Verification items for the finished model (mm, model axes). A direction names the side the tool comes from. Give positions to 0.01 mm unless a question says otherwise; leave off trailing zeros. Order: outer loops, then holes, each group sorted by start corner. A loop starts at its lowest first (then second) coordinate and runs counter-clockwise, first axis right, second up. Notation, with made-up numbers: (-24.5, 77) -> (15.5, 77) arc R10 cw to (15.5, 91) -> close; hole circle Ø11 at (-21.75, 83.25). An arc over 180 degrees is marked (long way). Return JSON: item names as keys, results as strings. Group by question number.
(1) Tool access check on faces 4 (the face through (-18, 0, 12.3)), 5 (the face through (-0.3, -18, 9.8)), 6 (the face through (0.3, 18, 9.8)). Record the directions out of +Z, -Z, +X, -X, +Y, -Y that give a thin tool (end or side, any length) a straight path to the whole face; none if there is none.
(2) Cross-section at C-C on x = 8. Enter the section's corners in (y, z).
(3) Depth check by flat-ended pin: pin 1 Ø5.5 at (x, y) = (6, 27) entering from -Z; pin 2 Ø3.5 at (x, y) = (-18, 7) entering from +Z; pin 3 Ø8.5 at (x, y) = (0, 0) entering from +Z; pin 4 Ø3 at (x, z) = (-10.5, 10) entering from -Y. Enter the tip coordinate at first touch or a pass-through.
(4) Thickness scan on line 1 along X through (y, z) = (0, 14.2); line 2 along X through (y, z) = (0, 9.55); line 3 along Y through (x, z) = (0, 13.1). Record the ranges inside material, lowest first.
(5) Cross-section at B-B on z = 15.5. Enter the section's corners in (x, y), then the cut area to 3 significant figures.
(6) Cross-section at A-A on x = 0. Enter the section's corners in (y, z).
(7) Release check for a two-part mould opening along Y. For faces 1 (the face through (0, -35, 14)), 2 (the face through (3, -2, 10.8)), 3 (the face through (15, 34, 14)) record: pulls with the +Y half, pulls with the -Y half, needs draft (parallel to the pull), parting line crosses it, or undercut.
Autodesk Fusion 360 part; units mm, degrees
ref_plane "工作平面1" through (0, 0, 12.3) normal (0, 0, 1) x (1, 0, 0)
sketch "草图1" plane through (0, 0, 12.3) normal (0, 0, 1) x (1, 0, 0)
  line L0 (-33, -16) -> (33, -16)
  line L1 (33, -16) -> (35, -14)
  line L2 (35, -14) -> (35, 14)
  line L3 (35, 14) -> (33, 16)
  line L4 (33, 16) -> (-33, 16)
  line L5 (-33, 16) -> (-35, 14)
  line L6 (-35, 14) -> (-35, -14)
  line L7 (-35, -14) -> (-33, -16)
extrude "70 x 32 camera support plate" add sketch "草图1" along normal blind 4
ref_plane "工作平面2" through (0, 0, 7.3) normal (0, 0, 1) x (1, 0, 0)
sketch "草图2" plane through (0, 0, 7.3) normal (0, 0, 1) x (1, 0, 0)
  line L0 (-20, -19) -> (20, -19)
  line L1 (20, -19) -> (20, 19)
  line L2 (20, 19) -> (-20, 19)
  line L3 (-20, 19) -> (-20, -19)
ref_plane "工作平面3" through (0, 0, 12.3) normal (0, 0, 1) x (1, 0, 0)
sketch "草图3" plane through (0, 0, 12.3) normal (0, 0, 1) x (1, 0, 0)
  line L0 (-16, -19) -> (16, -19)
  line L1 (16, -19) -> (16, 19)
  line L2 (16, 19) -> (-16, 19)
  line L3 (-16, 19) -> (-16, -19)
loft "40 to 32 mm male dovetail" add profiles "草图2", "草图3" section 1 section 2
ref_plane "工作平面4" through (0, 0, 7.3) normal (0, 0, 1) x (1, 0, 0)
sketch "草图4" plane through (0, 0, 7.3) normal (0, 0, 1) x (1, 0, 0)
  circle A0 centre (0, 0) radius 3.4
extrude "1/4 inch metal screw clearance 6.8 mm" cut sketch "草图4" along normal blind 9
ref_plane "工作平面5" through (0, 0, 7.3) normal (0, 0, 1) x (1, 0, 0)
sketch "草图5" plane through (0, 0, 7.3) normal (0, 0, 1) x (1, 0, 0)
  circle A0 centre (0, 0) radius 7
extrude "14 x 3.5 mm screw head recess" cut sketch "草图5" along normal blind 3.5
move_body "Align camera long edge with gimbal arm - 90 degrees" bodies 1 to x (0, 1, 0) y (-1, 0, 0) z (0, 0, 1) at (0, 0, 0)
Verdict:
{
 "1": {"face 4": "+Z, -X, +Y, -Y", "face 5": "+X, -X, -Y", "face 6": "+X, -X, +Y"},
 "2": {"outline": "(-35, 12.3) -> (-16, 12.3) -> (-20, 7.3) -> (20, 7.3) -> (16, 12.3) -> (35, 12.3) -> (35, 16.3) -> (-35, 16.3) -> close"},
 "3": {"pin 1": "z = 12.3", "pin 2": "z = 12.3", "pin 3": "z = 16.3", "pin 4": "y = -19.04"},
 "4": {"line 1": "-16 to -3.4, 3.4 to 16", "line 2": "-19 to -7, 7 to 19", "line 3": "-35 to -3.4, 3.4 to 35"},
 "5": {"outline": "(-16, -33) -> (-14, -35) -> (14, -35) -> (16, -33) -> (16, 33) -> (14, 35) -> (-14, 35) -> (-16, 33) -> close; hole circle Ø6.8 at (0, 0)", "area": "2,200 mm²"},
 "6": {"outline": "(-35, 12.3) -> (-16, 12.3) -> (-20, 7.3) -> (-7, 7.3) -> (-7, 10.8) -> (-3.4, 10.8) -> (-3.4, 16.3) -> (-35, 16.3) -> close; (3.4, 10.8) -> (7, 10.8) -> (7, 7.3) -> (20, 7.3) -> (16, 12.3) -> (35, 12.3) -> (35, 16.3) -> (3.4, 16.3) -> close"},
 "7": {"face 1": "pulls with the -Y half", "face 2": "undercut", "face 3": "pulls with the +Y half"}
}
